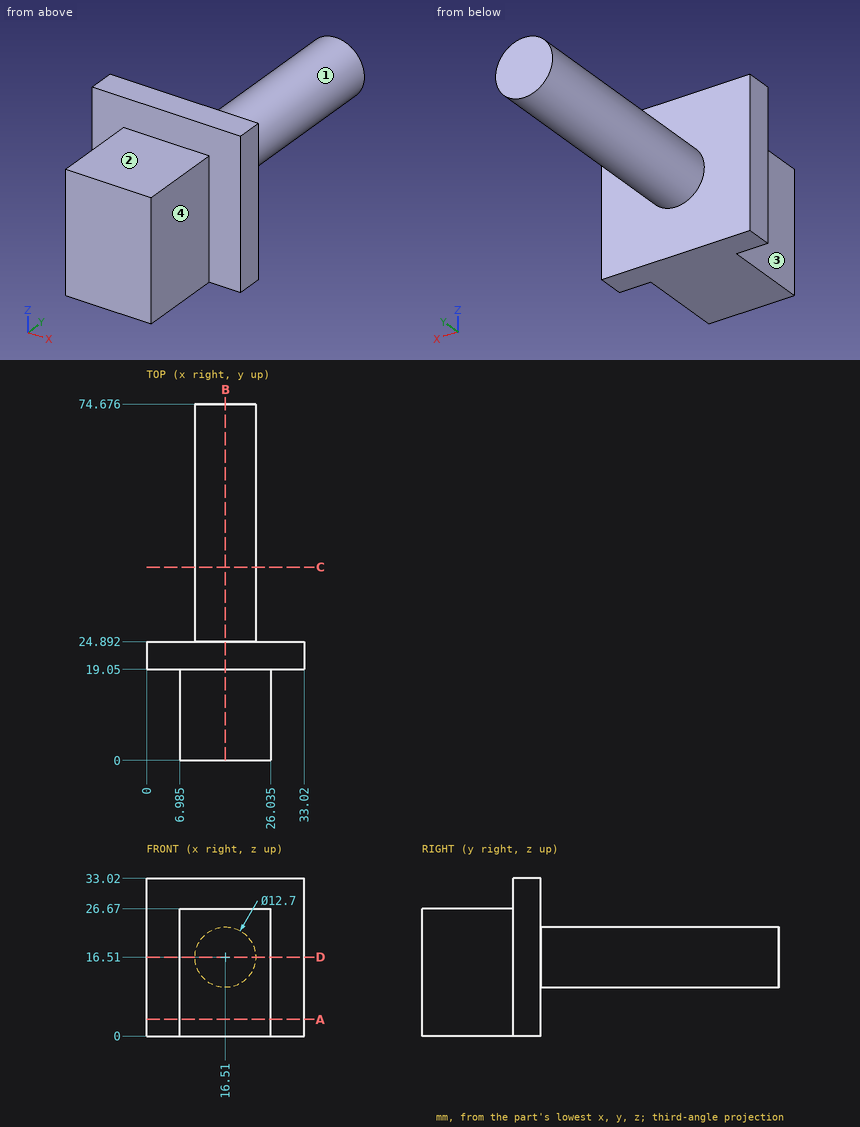
Verification items for this drawing (mm, ordinates from the low corner). A direction names the side the tool comes from. Give positions to 0.01 mm unless a question says otherwise; leave off trailing zeros. Loops run counter-clockwise (first coordinate to the right, second up) from the corner with the lowest first, then second, coordinate; pieces in that order, holes last.
1. Cross-section at A-A on z = 3.5. Record the cut outline in (x, y) (3 decimals).
Derived:
outline: (0, 19.05) - (6.985, 19.05) - (6.985, 0) - (26.035, 0) - (26.035, 19.05) - (33.02, 19.05) - (33.02, 24.892) - (0, 24.892) - close
2. Cross-section at C-C on y = 40.5. Record the cut outline in (x, z), and give its area (3 significant figures).
Derived:
outline: circle Ø12.7 at (16.51, 16.51)
area: 127 mm2
3. Go/stop test with flat-tipped pins: P1, Ø9.5, axis at y = 10.5, z = 13, coming from the +X side (3 decimals); P2, Ø1, axis at y = 61.5, z = 13, coming from the -X side; P3, Ø4, axis at x = 11.5, z = 24.5, coming from the +Y side. Record where each tip stops, or that it passes through.
Derived:
P1: stops at x = 26.035
P2: stops at x = 10.92
P3: stops at y = 24.89
4. Material ranges on probe 1 along Y at (x, z) = (8.5, 11.5); probe 2 along Y at (x, z) = (28, 10.5); probe 3 along X at (y, z) = (12, 19) (3 decimals), recorded low to high.
Derived:
probe 1: y = 0 to 24.89
probe 2: y = 19.05 to 24.89
probe 3: x = 6.985 to 26.035
5. Cross-section at D-D on z = 16.51. Record the cut outline in (x, y) (3 decimals), and give its area (3 significant figures).
Derived:
outline: (0, 19.05) - (6.985, 19.05) - (6.985, 0) - (26.035, 0) - (26.035, 19.05) - (33.02, 19.05) - (33.02, 24.892) - (22.86, 24.892) - (22.86, 74.676) - (10.16, 74.676) - (10.16, 24.892) - (0, 24.892) - close
area: 1,190 mm2
6. Tool access check on the marked faces 1, 2, 3 and 4. Record the directions out of +Z, -Z, +X, -X, +Y, -Y that give a thin tool (end or side, any length) a straight path to the whole face; none if there is none.
Derived:
face 1: +Y
face 2: +Z, +X, -X, -Y
face 3: +Z, -Z, -X, -Y
face 4: +Z, -Z, +X, -Y
7. Cross-section at B-B on x = 16.51. Record the cut outline in (y, z).
Derived:
outline: (0, 0) - (24.89, 0) - (24.89, 10.16) - (74.68, 10.16) - (74.68, 22.86) - (24.89, 22.86) - (24.89, 33.02) - (19.05, 33.02) - (19.05, 26.67) - (0, 26.67) - close
